```python
from build123d import *

# Parameters (mm, degrees)
F0_W     = 27
F0_H     = 151
F0_W_2   = 23
F0_H_2   = 145
F1_DEPTH = 27
F3_DEPTH = 2
F2_R     = 2
F4_DEPTH = 1
F5_W     = 27
F5_H     = 27
F5_R     = 8.5
F6_DEPTH = 25
F5_R_2   = 3.5
F7_DEPTH = 4
F8_SIZE  = 1


with BuildPart() as f1:
    # F0 (on Top) → F1 (new body)
    with BuildSketch(Plane.XY):
        with Locations((0, 71.5)):
            Rectangle(F0_W, F0_H)
        with Locations((0, 72.5)):
            Rectangle(F0_W_2, F0_H_2, mode=Mode.SUBTRACT)
    extrude(amount=F1_DEPTH)

    # F0 (on Top) → F3 (join)
    with BuildSketch(Plane.XY):
        with Locations((0, 72.5)):
            Rectangle(F0_W_2, F0_H_2)
    extrude(amount=F3_DEPTH)

    # F2 (on face) → F4 (cut)
    with BuildSketch(Plane(origin=(0, 147, 0), x_dir=(-1, 0, 0), z_dir=(0, 1, 0))):
        with Locations((0, 5.5)):
            Circle(F2_R)
    extrude(amount=-F4_DEPTH, mode=Mode.SUBTRACT)

    # F5 (on face) → F6 (join)
    with BuildSketch(Plane.XZ.offset(4)):
        with Locations((0, 13.5)):
            Rectangle(F5_W, F5_H)
        with Locations((0, 13.5)):
            Circle(F5_R, mode=Mode.SUBTRACT)
    extrude(amount=F6_DEPTH)

    # F5 (on face) → F7 (cut, through all)
    with BuildSketch(Plane.XZ.offset(4)):
        with Locations((2.2, 17.5)):
            Circle(F5_R_2)
    extrude(amount=-F7_DEPTH, mode=Mode.SUBTRACT)

    # F8
    f8_edges = [f1.edges().sort_by_distance(p)[0] for p in [
        (-8.5, -29, 13.5),
    ]]
    chamfer(f8_edges, length=F8_SIZE)


solid = f1.part
```
Part model, mm, in its own coordinate system. A direction names the side the tool comes from. Coordinates: 2 decimals unless noted, no trailing zeros. Order: outer loops, then holes, each group sorted by start corner. A loop starts at its lowest first (then second) coordinate and runs counter-clockwise, first axis right, second up. Notation, with made-up numbers: (30, 55.5) - (61, 55.5) arc R30 cw to (61, 81.5) - close; hole circle Ø6 at (63.5, 6.25). An arc over 180 degrees is marked (long way). Return JSON: item names as keys, results as strings. Group by question number.
Item 1: Cut at A-A (y = -13). List the corners of the cut face in (x, z).
Item 2: Pull direction Z, two halves, no side cores. Call faces 5 (the face through (0, -4, 13)), 6 (the face through (0, 145, 14)), 7 (the face through (0, 60, 0)): pulls with the +Z half, pulls with the -Z half, needs draft (parallel to the pull), parting line crosses it, or undercut.
Item 3: Drill centre lines: probe 1 along Y at (x, z) = (-3.75, 9.75); probe 2 along Z at (x, y) = (0, -23); probe 3 along X at (y, z) = (6, 13). Where is each one in solid material? Low to high. Write a range as from..to.
Item 4: Which spindle directions (+Z, -Z, +X, -X, +Y, -Y) get a long thin tool onto all of the face, cutting with end or side? Do faces 1 (the face through (0, 146, 6)), 2 (the face through (-3, -29, 23)), 3 (the face through (-1.84, -15.83, 5.2)), 4 (the face through (0, 74, 2)). Say none if no direction does.
Item 5: Pin check, flat tips, straight feed: pin 1 (4 mm diameter, centred on x = 2.2, z = 17.5, fed in from -Y); pin 2 (7 mm diameter, centred on x = -5.5, y = 50, fed in from +Z); pin 3 (1 mm diameter, centred on x = -3.5, z = 14.5, fed in from -Y). Stop position of each tip, or through.
Item 6: Cut at B-B (y = 85). List the corners of the cut face in (x, z), plus the area to 3 significant figures.
Check values:
{
 "1": {"outline": "(-13.5, 0) - (13.5, 0) - (13.5, 27) - (-13.5, 27) - close; hole circle Ø17 at (0, 13.5)"},
 "2": {"face 5": "undercut", "face 6": "needs draft", "face 7": "pulls with the -Z half"},
 "3": {"probe 1": "y = -4..0, 145..147", "probe 2": "z = 0..5, 22..27", "probe 3": "x = -13.5..-11.5, 11.5..13.5"},
 "4": {"face 1": "+Y", "face 2": "+Z, -Z, +X, -X, -Y", "face 3": "-Y", "face 4": "+Z"},
 "5": {"pin 1": "stops at y = 145", "pin 2": "stops at z = 2", "pin 3": "stops at y = -4"},
 "6": {"outline": "(-13.5, 0) - (13.5, 0) - (13.5, 27) - (11.5, 27) - (11.5, 2) - (-11.5, 2) - (-11.5, 27) - (-13.5, 27) - close", "area": "154 mm2"}
}
